Drawing for the job (mm, zero at the part's lowest x, y, z). A direction names the side the tool comes from. Give positions to 0.01 mm unless a question says otherwise; leave off trailing zeros. Order: outer loops, then holes, each group sorted by start corner. A loop starts at its lowest first (then second) coordinate and runs counter-clockwise, first axis right, second up. Notation, with made-up numbers: (84, -35) -> (134, -35) arc R19 cw to (134, -5) -> close; hole circle Ø7 at (-29, 4). An arc over 180 degrees is marked (long way). One line per item, written item: value. Start each with the question number.
(1) Saw through at A-A on z = 49. Give the cut face in (x, y) (3 decimals).
(2) Saw through at D-D on x = 44.45. Give the cut face in (y, z) (3 decimals), plus the area to 3 significant figures.
(3) Saw through at B-B on y = 43.5. Give the cut face in (x, z) (3 decimals).
(4) Probe line 1 (X direction, y = 55.5, z = 17) (3 decimals); line 2 (Z direction, x = 7, y = 46) (3 decimals); line 3 (X direction, y = 26, z = 66.5). List the from-to ranges inside material, lowest first.
(5) Saw through at C-C on x = 63. Give the cut face in (y, z) (3 decimals).
(6) Pin check, flat tip, straight feed: pin 1 (3 mm diameter, centred on x = 22.5, y = 25.5, fed in from -Z). Stop position of the tip, or through.
(7) Which spindle directions (+Z, -Z, +X, -X, +Y, -Y) get a long thin tool onto all of the face, cutting with end or side? Do the marked faces 1 and 2. Say none if no direction does.
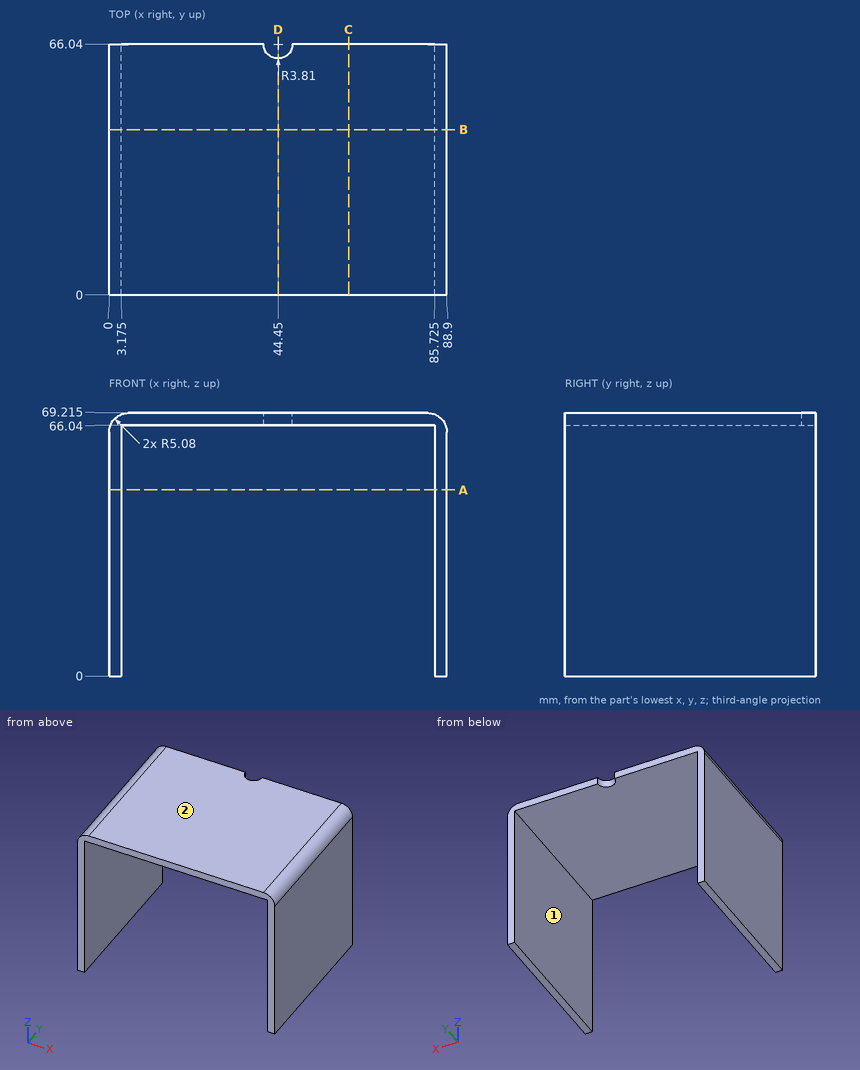
Results below:
1. outline: (0, 0) -> (3.175, 0) -> (3.175, 66.04) -> (0, 66.04) -> close; (85.725, 0) -> (88.9, 0) -> (88.9, 66.04) -> (85.725, 66.04) -> close
2. outline: (0, 66.04) -> (62.23, 66.04) -> (62.23, 69.215) -> (0, 69.215) -> close
2. area: 198 mm²
3. outline: (0, 0) -> (3.175, 0) -> (3.175, 66.04) -> (85.725, 66.04) -> (85.725, 0) -> (88.9, 0) -> (88.9, 64.135) arc R5.08 ccw to (83.82, 69.215) -> (5.08, 69.215) arc R5.08 ccw to (0, 64.135) -> close
4. line 1: x = 0 to 3.175, 85.725 to 88.9
4. line 2: z = 66.04 to 69.215
4. line 3: x = 0.58 to 88.32
5. outline: (0, 66.04) -> (66.04, 66.04) -> (66.04, 69.215) -> (0, 69.215) -> close
6. pin 1: stops at z = 66.04
7. face 1: -Z, +Y, -Y
7. face 2: +Z, +X, -X, +Y, -Y
